from build123d import *

# Parameters (mm, degrees)
SKETCH1_R           = 4.5
BOSS_EXTRUDE1_DEPTH = 10.25
SKETCH3_R           = 2.55
CUT_EXTRUDE1_DEPTH  = 34
BOSS_EXTRUDE2_START = -4
SKETCH4_R           = 8
SKETCH4_R_2         = 4.5
BOSS_EXTRUDE2_DEPTH = 4
FILLET1_R           = 2.5
FILLET2_R           = 2.5
SKETCH5_R           = 3
SKETCH5_R_2         = 2.55
CUT_EXTRUDE2_DEPTH  = 0.7


with BuildPart() as part:
    # Sketch1 → Boss-Extrude1 (new body)
    with BuildSketch(Plane(origin=(0, 0, 0), x_dir=(0, 0, -1), z_dir=(1, 0, 0))):
        Circle(SKETCH1_R)
    extrude(amount=BOSS_EXTRUDE1_DEPTH)

    # Sketch3 → Cut-Extrude1 (cut)
    with BuildSketch(Plane.ZY):
        Circle(SKETCH3_R)
    extrude(amount=-CUT_EXTRUDE1_DEPTH, mode=Mode.SUBTRACT)

    # Sketch4 → Boss-Extrude2 (add)
    with BuildSketch(Plane(origin=(10.25, 0, 0), x_dir=(0, 0, -1), z_dir=(1, 0, 0)).offset(BOSS_EXTRUDE2_START)):
        Circle(SKETCH4_R)
        Circle(SKETCH4_R_2, mode=Mode.SUBTRACT)
    extrude(amount=BOSS_EXTRUDE2_DEPTH)

    # Fillet1
    fillet1_edges = [part.edges().sort_by_distance(p)[0] for p in [
        (6.25, 0, 8),
    ]]
    fillet(fillet1_edges, radius=FILLET1_R)

    # Fillet2
    fillet2_edges = [part.edges().sort_by_distance(p)[0] for p in [
        (6.25, 0, 4.5),
    ]]
    fillet(fillet2_edges, radius=FILLET2_R)

    # Sketch5 → Cut-Extrude2 (cut)
    with BuildSketch(Plane.ZY):
        Circle(SKETCH5_R)
        Circle(SKETCH5_R_2, mode=Mode.SUBTRACT)
    extrude(amount=-CUT_EXTRUDE2_DEPTH, mode=Mode.SUBTRACT)


solid = part.part
Can you work these out from the model? Positions are in its coordinate system, mm. A direction names the side the tool comes from. Round coordinates to 2 decimals unless told otherwise and drop trailing zeros. Order: outer loops, then holes, each group sorted by start corner. A loop starts at its lowest first (then second) coordinate and runs counter-clockwise, first axis right, second up. Notation, with made-up numbers: M 47,89 L 100,89 A11 ccw 100,95 Z; hole C 34,19.5 d4. An arc over 180 degrees is marked long. Use a Markdown table: item, result.
1) Imagine slicing it at B-B (x = 7.75). List the corners of the cut face in (y, z) for me.
Geometry says:
| item | result |
|---|---|
| outline | C 0,0 d15.58; hole C 0,0 d5.1 |
2) On a 3-axis mill with a long thin cutter (end or side, diameter ignored), from which of +Z, -Z, +X, -X, +Y, -Y can I reach the whole of each face in a straight line? I mean faces 1 (the face through (10.25, 2, 2)), 2 (the face through (0.7, 2, -2)). Say none if no direction works.
Geometry says:
| item | result |
|---|---|
| face 1 | +Z, -Z, +X, +Y, -Y |
| face 2 | -X |
3) Imagine slicing it at A-A (x = 9.5). List the corners of the cut face in (y, z) for me, then the cut area to 3 significant figures.
Geometry says:
| item | result |
|---|---|
| outline | C 0,0 d16; hole C 0,0 d5.1 |
| area | 181 mm² |
4) If I drill on line 1 along Y through (x, z) = (0.5, 0); line 2 along X through (y, z) = (2.75, -0.5); line 3 along Z through (x, y) = (8, -1), over which ranges is the centre line in solid material (lowest first)?
Geometry says:
| item | result |
|---|---|
| line 1 | y = -4.5 to -3, 3 to 4.5 |
| line 2 | x = 0.7 to 10.25 |
| line 3 | z = -7.82 to -2.35, 2.35 to 7.82 |
5) I'm going to push flat-ended pins straight in: P1, Ø3, axis at x = 3.5, z = 5, coming from the -Y side; P2, Ø2, axis at x = 8, z = -3, coming from the +Y side; P3, Ø1.5, axis at x = 6.5, y = -3.5, coming from the -Z side; P4, Ø4, axis at y = 0, z = 0, coming from the -X side. Where does each tip first touch, or does it pass through?
Geometry says:
| item | result |
|---|---|
| P1 | stops at y = -2.83 |
| P2 | stops at y = 7.7 |
| P3 | stops at z = -6.73 |
| P4 | passes through |
